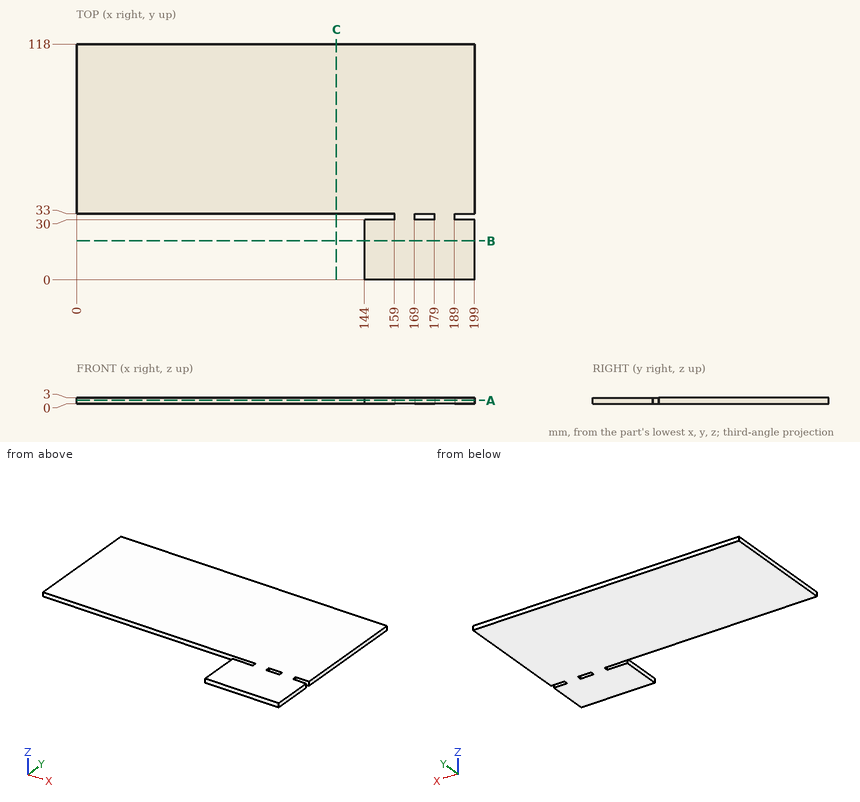
For this review, use the dimensioned drawing (mm, ordinates from the lowest corner) and the shaded views. Coordinates: 2 decimals unless noted, no trailing zeros. Write each loop counter-clockwise with the first axis right and the second up, starting at its lowest first coordinate (ties: lowest second). Pieces come first, ordered by that corner, then holes. Notation, with made-up numbers: (-25.75, 80.5) - (15.25, 80.5) arc R28 cw to (15.25, 113.5) - close; hole circle Ø2 at (3, 85). An arc over 180 degrees is marked (long way). Answer as a JSON object with one key per item and string values. Group by question number.
1. Add section A-A (z = 1.8). Give the boundary of the cut face in (x, y).
2. Add section B-B (y = 19.5). Give the boundary of the cut face in (x, z), plus the area to 3 significant figures.
3. Add section C-C (x = 130). Give the boundary of the cut face in (y, z), plus the area to 3 significant figures.
4. Clearance check with flat-ended pins moving along their axes: pin 1 Ø1.5 at (y, z) = (32, 1.5) entering from -X; pin 2 Ø1.5 at (y, z) = (32, 1) entering from +X; pin 3 Ø1.5 at (x, z) = (107.5, 2) entering from -Y. State where each tip first meets the part, or that it passes through.
5. To check wall thickness, follow probe 1 along Y at (x, z) = (176, 0.55); probe 2 along X at (y, z) = (12.5, 0.8); probe 3 along Y at (x, z) = (90, 1.4). State the ranges of each line that lie inside material, in increasing order.
Findings:
{
 "1": {"outline": "(0, 33) - (159, 33) - (159, 30) - (144, 30) - (144, 0) - (199, 0) - (199, 30) - (189, 30) - (189, 33) - (199, 33) - (199, 118) - (0, 118) - close; hole (169, 30) - (179, 30) - (179, 33) - (169, 33) - close"},
 "2": {"outline": "(144, 0) - (199, 0) - (199, 3) - (144, 3) - close", "area": "165 mm²"},
 "3": {"outline": "(33, 0) - (118, 0) - (118, 3) - (33, 3) - close", "area": "255 mm²"},
 "4": {"pin 1": "x = 159", "pin 2": "x = 189", "pin 3": "y = 33"},
 "5": {"probe 1": "0 to 30, 33 to 118", "probe 2": "144 to 199", "probe 3": "33 to 118"}
}
